Job drawing, mm, ordinate dimensions from the low corner. One solid piece. Round coordinates to 2 decimals unless told otherwise and drop trailing zeros. Loops run counter-clockwise (first coordinate to the right, second up) from the corner with the lowest first, then second, coordinate; pieces in that order, holes last.
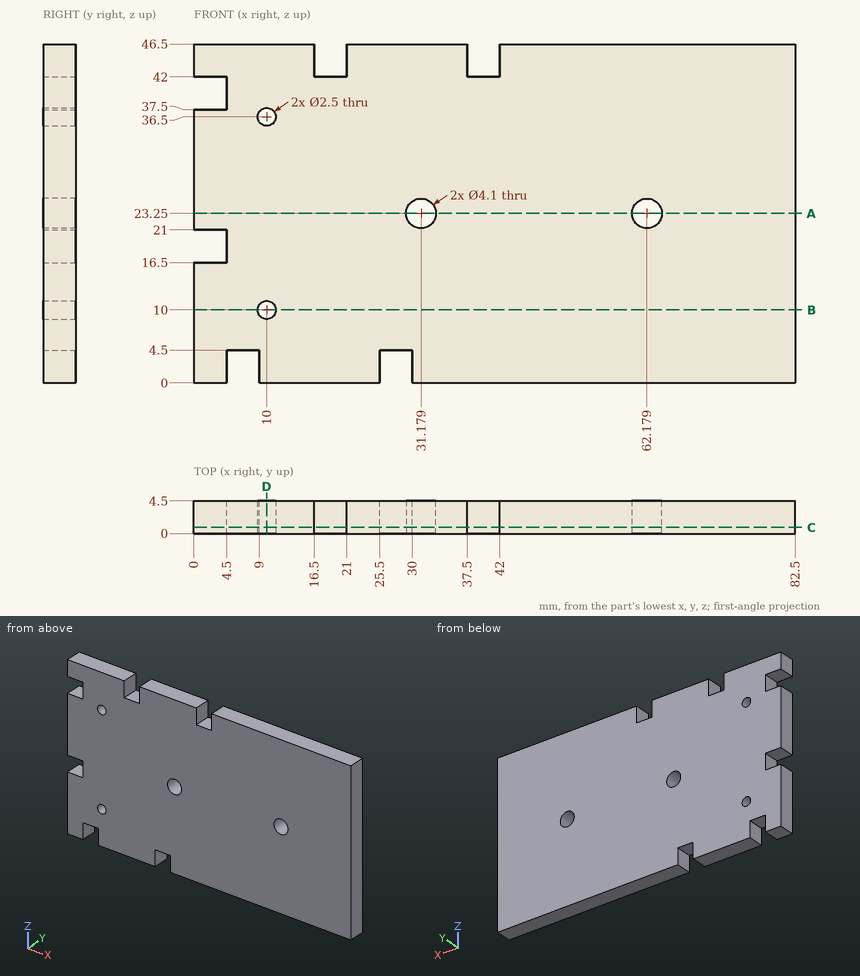
1) Slice it at A-A, the plane z = 23.25. Give the cut face in (x, y), then the cut area to 3 significant figures.
Values:
outline: (0, 0) - (29.13, 0) - (29.13, 4.5) - (0, 4.5) - close; (33.23, 0) - (60.13, 0) - (60.13, 4.5) - (33.23, 4.5) - close; (64.23, 0) - (82.5, 0) - (82.5, 4.5) - (64.23, 4.5) - close
area: 334 mm2
2) Slice it at C-C, the plane y = 0.85. Give the number of separate pieces and of enclosed holes in the cut face, then the cut area to 3 significant figures.
Values:
separate pieces: 1
enclosed holes: 4
area: 3,680 mm2
3) Drop flat-ended pins along their axis: pin 1 Ø2 at (x, y) = (6, 2) entering from -Z; pin 2 Ø1.5 at (y, z) = (0.5, 20) entering from -X. Give the stop position or say it passes through.
Values:
pin 1: stops at z = 4.5
pin 2: stops at x = 4.5
4) Slice it at D-D, the plane x = 10. Give the cut face in (y, z).
Values:
outline: (0, 0) - (4.5, 0) - (4.5, 8.75) - (0, 8.75) - close; (0, 11.25) - (4.5, 11.25) - (4.5, 35.25) - (0, 35.25) - close; (0, 37.75) - (4.5, 37.75) - (4.5, 46.5) - (0, 46.5) - close
5) Slice it at B-B, the plane z = 10. Give the cut face in (x, y).
Values:
outline: (0, 0) - (8.75, 0) - (8.75, 4.5) - (0, 4.5) - close; (11.25, 0) - (82.5, 0) - (82.5, 4.5) - (11.25, 4.5) - close
6) Wall check: line 1 along X through (y, z) = (0.7, 44); line 2 along X through (y, z) = (3.75, 2.5); line 3 along Z through (x, y) = (10, 3.35). Give the ranges that are in metal, low to high.
Values:
line 1: x = 0 to 16.5, 21 to 37.5, 42 to 82.5
line 2: x = 0 to 4.5, 9 to 25.5, 30 to 82.5
line 3: z = 0 to 8.75, 11.25 to 35.25, 37.75 to 46.5
